from build123d import *

# Parameters (mm, degrees)
CROQUIS1_R              = 2.1
SALIENTE_EXTRUIR2_DEPTH = 100


with BuildPart() as part:
    # Croquis1 → Saliente-Extruir2 (new body)
    with BuildSketch(Plane(origin=(0, 0, 0), x_dir=(1, 0, 0), z_dir=(0, 1, 0))):
        with BuildLine():
            Line((3.9, -2.84), (3.9, 2.84))
            Line((3.9, 2.84), (6.36, 5.3))
            Line((6.36, 5.3), (8.2, 5.3))
            Line((8.2, 5.3), (8.2, 3.34))
            ThreePointArc((8.2, 3.34), (8.346446609, 2.986446609), (8.7, 2.84))
            Line((8.7, 2.84), (10, 4.14))
            Line((10, 4.14), (10, 8))
            ThreePointArc((10, 8), (9.414213562, 9.414213562), (8, 10))
            Line((8, 10), (4.14, 10))
            Line((4.14, 10), (2.84, 8.7))
            ThreePointArc((2.84, 8.7), (2.986446609, 8.346446609), (3.34, 8.2))
            Line((3.34, 8.2), (5.3, 8.2))
            Line((5.3, 8.2), (5.3, 6.36))
            Line((5.3, 6.36), (2.84, 3.9))
            Line((2.84, 3.9), (-2.84, 3.9))
            Line((-2.84, 3.9), (-5.3, 6.36))
            Line((-5.3, 6.36), (-5.3, 8.2))
            Line((-5.3, 8.2), (-3.34, 8.2))
            ThreePointArc((-3.34, 8.2), (-2.986446609, 8.346446609), (-2.84, 8.7))
            Line((-2.84, 8.7), (-4.14, 10))
            Line((-4.14, 10), (-8, 10))
            ThreePointArc((-8, 10), (-9.414213562, 9.414213562), (-10, 8))
            Line((-10, 8), (-10, 4.14))
            Line((-10, 4.14), (-8.7, 2.84))
            ThreePointArc((-8.7, 2.84), (-8.346446609, 2.986446609), (-8.2, 3.34))
            Line((-8.2, 3.34), (-8.2, 5.3))
            Line((-8.2, 5.3), (-6.36, 5.3))
            Line((-6.36, 5.3), (-3.9, 2.84))
            Line((-3.9, 2.84), (-3.9, -2.84))
            Line((-3.9, -2.84), (-6.36, -5.3))
            Line((-6.36, -5.3), (-8.2, -5.3))
            Line((-8.2, -5.3), (-8.2, -3.34))
            ThreePointArc((-8.2, -3.34), (-8.346446609, -2.986446609), (-8.7, -2.84))
            Line((-8.7, -2.84), (-10, -4.14))
            Line((-10, -4.14), (-10, -8))
            ThreePointArc((-10, -8), (-9.414213562, -9.414213562), (-8, -10))
            Line((-8, -10), (-4.14, -10))
            Line((-4.14, -10), (-2.84, -8.7))
            ThreePointArc((-2.84, -8.7), (-2.986446609, -8.346446609), (-3.34, -8.2))
            Line((-3.34, -8.2), (-5.3, -8.2))
            Line((-5.3, -8.2), (-5.3, -6.36))
            Line((-5.3, -6.36), (-2.84, -3.9))
            Line((-2.84, -3.9), (2.84, -3.9))
            Line((2.84, -3.9), (5.3, -6.36))
            Line((5.3, -6.36), (5.3, -8.2))
            Line((5.3, -8.2), (3.34, -8.2))
            ThreePointArc((3.34, -8.2), (2.986446609, -8.346446609), (2.84, -8.7))
            Line((2.84, -8.7), (4.14, -10))
            Line((4.14, -10), (8, -10))
            ThreePointArc((8, -10), (9.414213562, -9.414213562), (10, -8))
            Line((10, -8), (10, -4.14))
            Line((10, -4.14), (8.7, -2.84))
            ThreePointArc((8.7, -2.84), (8.346446609, -2.986446609), (8.2, -3.34))
            Line((8.2, -3.34), (8.2, -5.3))
            Line((8.2, -5.3), (6.36, -5.3))
            Line((6.36, -5.3), (3.9, -2.84))
        make_face()
        Circle(CROQUIS1_R, mode=Mode.SUBTRACT)
    extrude(amount=SALIENTE_EXTRUIR2_DEPTH)


solid = part.part
Verification items for the finished model (mm, model axes). A direction names the side the tool comes from. Give positions to 0.01 mm unless a question says otherwise; leave off trailing zeros. Write each loop counter-clockwise with the first axis right and the second up, starting at its lowest first coordinate (ties: lowest second). Pieces come first, ordered by that corner, then holes. Notation, with made-up numbers: M 5,-23 L 36,-23 A25 ccw 36,13 Z; hole C 84.5,40 d8. An arc over 180 degrees is marked long. Put each result on its own line as item: value. Start each with the question number.
1. Set-up check for faces 1 (the face through (-8.2, 49, 4)), 2 (the face through (10, 49, -6)), 3 (the face through (0, 49, -3.9)), 4 (the face through (-3.9, 49, 0)), 5 (the face through (3.9, 49, 0)): record each of +Z, -Z, +X, -X, +Y, -Y from which the full face is reachable in a straight line by a thin tool's end or side.
2. Scan lines: line 1 along X through (y, z) = (76.5, 0); line 2 along X through (y, z) = (20.5, -6.5). Record each from-to range of solid material in increasing order. Write a range as [from, to].
3. Draft check along Z on faces 6 (the face through (6, 49, 10)), 7 (the face through (7, 49, 5.3)), 8 (the face through (10, 49, 6)). Enter one of: +Z half, -Z half, draft (parallel to the pull), parting line (faces both ways), or undercut.
4. Go/stop test with flat-tipped pins: pin 1 Ø3 at (y, z) = (38, 0.5) entering from +X; pin 2 Ø4.5 at (x, y) = (0.5, 45.5) entering from -Z; pin 3 Ø1.7 at (y, z) = (47, 1.5) entering from -X. Record where each tip stops, or that it passes through.
5. Section check A-A (x = 0). Record the cut outline in (y, z).
6. Section check B-B (z = 0). Record the cut outline in (x, y), and give its area (3 significant figures).
Answer list:
1. face 1: +Y, -Y
1. face 2: +Z, -Z, +X, +Y, -Y
1. face 3: -Z, +Y, -Y
1. face 4: -X, +Y, -Y
1. face 5: +X, +Y, -Y
2. line 1: [-3.9, -2.1], [2.1, 3.9]
2. line 2: [-10, -5.3], [5.3, 10]
3. face 6: +Z half
3. face 7: undercut
3. face 8: draft
4. pin 1: x = 3.9
4. pin 2: z = -3.9
4. pin 3: x = -3.9
5. outline: M 0,-3.9 L 100,-3.9 L 100,-2.1 L 0,-2.1 Z; M 0,2.1 L 100,2.1 L 100,3.9 L 0,3.9 Z
6. outline: M -3.9,0 L -2.1,0 L -2.1,100 L -3.9,100 Z; M 2.1,0 L 3.9,0 L 3.9,100 L 2.1,100 Z
6. area: 360 mm2
